Geometry: final body of the model. Coordinates: model frame, mm. Face numbers are marked on the shaded views. A direction names the side the tool comes from. Round coordinates to 2 decimals unless told otherwise and drop trailing zeros. Loops run counter-clockwise (first coordinate to the right, second up) from the corner with the lowest first, then second, coordinate; pieces in that order, holes last. Notation, with made-up numbers: (20.5, 51) - (54.5, 51) arc R23 ccw to (54.5, 71) - close; hole circle Ø9 at (-20.5, 60). An arc over 180 degrees is marked (long way). Answer in a Markdown table with one row per item. Add a question column.
from build123d import *

# Parameters (mm, degrees)
PAD_DEPTH         = 60
PAD_DEPTH_BACK    = 53
SKETCH001_R       = 11.1
SKETCH001_R_2     = 3.1
SKETCH001_R_3     = 1.6
SKETCH001_W       = 34.5
SKETCH001_H       = 60
POCKET_DEPTH      = 27.001
POCKET_DEPTH_BACK = -5.001
POCKET001_DEPTH   = 43.001
PAD001_DEPTH      = 5
PAD002_DEPTH      = 5
SKETCH005_W       = 43
SKETCH005_H       = 27
POCKET002_DEPTH   = 43.001
SKETCH006_W       = 5
SKETCH006_H       = 32
PAD003_DEPTH      = 15
SKETCH007_R       = 3.1
POCKET003_DEPTH   = 43.001
FILLET_R          = 2


with BuildPart() as part:
    # Sketch → Pad (new body, two sides)
    with BuildSketch(Plane.XZ) as pad_sk:
        Polygon((-43, 5), (27, 5), (27, 0), (0, 0), (0, -27), (-8.5, -27), (-8.5, 0), (-43, 0), align=None)
    extrude(amount=PAD_DEPTH)
    extrude(pad_sk.sketch, amount=-PAD_DEPTH_BACK)

    # Sketch001 → Pocket (cut, two sides)
    with BuildSketch(Plane.XY) as pocket_sk:
        with Locations((-22, 26.5)):
            Circle(SKETCH001_R)
        with Locations((15, 42)):
            Circle(SKETCH001_R_2)
        with Locations((15, -42)):
            Circle(SKETCH001_R_2)
        with Locations((15, 0)):
            Circle(SKETCH001_R_2)
        with Locations((-37.5, 42)):
            Circle(SKETCH001_R_3)
        with Locations((-6.5, 42)):
            Circle(SKETCH001_R_3)
        with Locations((-6.5, 11)):
            Circle(SKETCH001_R_3)
        with Locations((-37.5, 11)):
            Circle(SKETCH001_R_3)
        with Locations((-25.75, -30)):
            Rectangle(SKETCH001_W, SKETCH001_H)
    extrude(amount=-POCKET_DEPTH, mode=Mode.SUBTRACT)
    extrude(pocket_sk.sketch, amount=-POCKET_DEPTH_BACK, mode=Mode.SUBTRACT)

    # Sketch002 → Pocket001 (cut, through all)
    with BuildSketch(Plane.YZ):
        with BuildLine():
            ThreePointArc((-52.5, -11.9), (-55.6, -15), (-52.5, -18.1))
            Line((-52.5, -18.1), (-49.5, -18.1))
            ThreePointArc((-49.5, -18.1), (-46.4, -15), (-49.5, -11.9))
            Line((-52.5, -11.9), (-49.5, -11.9))
        make_face()
        with BuildLine():
            ThreePointArc((-10.5, -11.9), (-13.6, -15), (-10.5, -18.1))
            Line((-10.5, -18.1), (-7.5, -18.1))
            ThreePointArc((-7.5, -18.1), (-4.4, -15), (-7.5, -11.9))
            Line((-10.5, -11.9), (-7.5, -11.9))
        make_face()
    extrude(amount=-POCKET001_DEPTH, mode=Mode.SUBTRACT)

    # Sketch003 → Pad001 (join)
    with BuildSketch(Plane.XZ):
        Polygon((-43, 5), (-43, 0), (-8.5, -27), (0, -27), (0, 5), align=None)
    extrude(amount=-PAD001_DEPTH)

    # Sketch004 (on Face1 of Pad001) → Pad002 (join)
    with BuildSketch(Plane(origin=(0, 53, 0), x_dir=(1, 0, 0), z_dir=(0, 1, 0))):
        Polygon((-43, -5), (0, -5), (0, 27), (-8.5, 27), (-43, 0), align=None)
    extrude(amount=-PAD002_DEPTH)

    # Sketch005 → Pocket002 (cut, through all)
    with BuildSketch(Plane.YZ):
        with Locations((26.5, -13.5)):
            Rectangle(SKETCH005_W, SKETCH005_H)
    extrude(amount=-POCKET002_DEPTH, mode=Mode.SUBTRACT)

    # Sketch006 (on Face4 of Pocket002) → Pad003 (join)
    with BuildSketch(Plane(origin=(0, 53, 0), x_dir=(1, 0, 0), z_dir=(0, 1, 0))):
        with Locations((-2.5, 11)):
            Rectangle(SKETCH006_W, SKETCH006_H)
    extrude(amount=PAD003_DEPTH)

    # Sketch007 → Pocket003 (cut, through all)
    with BuildSketch(Plane.YZ):
        with Locations((60.5, -15)):
            Circle(SKETCH007_R)
    extrude(amount=-POCKET003_DEPTH, mode=Mode.SUBTRACT)

    # Fillet
    fillet_edges = [part.edges().sort_by_distance(p)[0] for p in [
        (27, -60, 2.5),
        (27, 53, 2.5),
        (-43, 0, 2.5),
        (-43, 53, 2.5),
    ]]
    fillet(fillet_edges, radius=FILLET_R)


solid = part.part
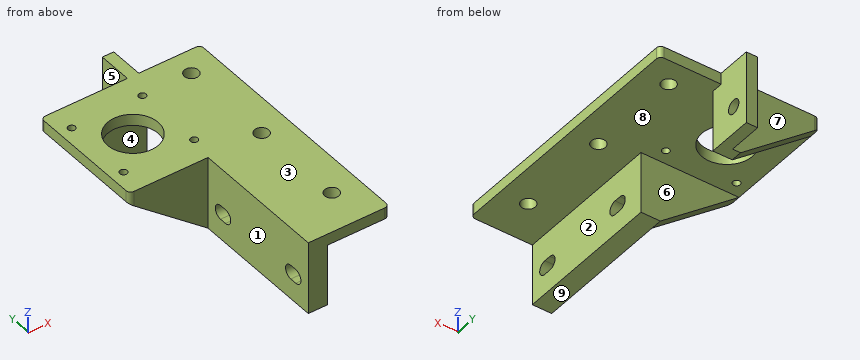
1) Contact query for flat-ended pins moving along their axis: pin 1 Ø9.5 at (x, z) = (-16.5, -18.5) entering from -Y; pin 2 Ø10 at (y, z) = (60.5, -15) entering from -X; pin 3 Ø6 at (y, z) = (59.5, -13) entering from +X. Output: stop coordinate, or through.
2) Section D-D, the plane y = 11. Return the cut outline in (x, z), and give its area (3 significant figures).
3) Section C-C, the plane x = -24.5. Return the cut outline in (y, z), and give its area (3 significant figures).
4) Material intervals for line 1 along Y through (x, z) = (15, 3); line 2 along Y through (x, z) = (-6.5, 2.85); line 3 along Y through (x, z) = (-37.5, 1.75), sorted ascending. Write a range as from..to.
5) Reachability of the marked faces 1, 2, 3, 4 and 5 from +Z, -Z, +X, -X, +Y, -Y: full face, straight path, thin tool, end or side. Return the list, or none.
6) Section B-B, the plane z = -15. Return the cut outline in (x, y).
7) Pull-direction query (Y, two-part tool) for the marked faces 6, 7, 8 and 9; classes: pulls with the +Y half, pulls with the -Y half, needs draft (parallel to the pull), parting line crosses it, or undercut.
8) Section A-A, the plane y = 26.5. Return the cut outline in (x, z), and give its area (3 significant figures).
Evaluation:
| question | item | result |
|---|---|---|
| 1 | pin 1 | stops at y = 0 |
| 1 | pin 2 | stops at x = -5 |
| 1 | pin 3 | stops at x = 0 |
| 2 | outline | (-43, 0) - (-39.1, 0) - (-39.1, 5) - (-43, 5) - close; (-35.9, 0) - (-8.1, 0) - (-8.1, 5) - (-35.9, 5) - close; (-4.9, 0) - (27, 0) - (27, 5) - (-4.9, 5) - close |
| 2 | area | 318 mm² |
| 3 | outline | (0, -14.48) - (5, -14.48) - (5, 0) - (15.69, 0) - (15.69, 5) - (0, 5) - close; (37.31, 0) - (48, 0) - (48, -14.48) - (53, -14.48) - (53, 5) - (37.31, 5) - close |
| 3 | area | 302 mm² |
| 4 | line 1 | y = -60..-45.1, -38.9..-3.1, 3.1..38.9, 45.1..53 |
| 4 | line 2 | y = -60..9.4, 12.6..40.4, 43.6..53 |
| 4 | line 3 | y = 0..9.4, 12.6..40.4, 43.6..53 |
| 5 | face 1 | +Z, -Z, -X, -Y |
| 5 | face 2 | -Z, +X, +Y, -Y |
| 5 | face 3 | +Z, +X, -X, +Y, -Y |
| 5 | face 4 | -Z, +X, -X |
| 5 | face 5 | +Z, -Z, -X, +Y |
| 6 | outline | (-23.83, 0) - (-8.5, 0) - (-8.5, -4.4) - (0, -4.4) - (0, 5) - (-23.83, 5) - close; (-23.83, 48) - (0, 48) - (0, 57.4) - (-5, 57.4) - (-5, 53) - (-23.83, 53) - close; (-8.5, -60) - (0, -60) - (0, -55.6) - (-8.5, -55.6) - close; (-8.5, -46.4) - (0, -46.4) - (0, -13.6) - (-8.5, -13.6) - close; (-5, 63.6) - (0, 63.6) - (0, 68) - (-5, 68) - close |
| 7 | face 6 | undercut |
| 7 | face 7 | pulls with the +Y half |
| 7 | face 8 | undercut |
| 7 | face 9 | needs draft |
| 8 | outline | (-43, 0) - (-33.1, 0) - (-33.1, 5) - (-43, 5) - close; (-10.9, 0) - (27, 0) - (27, 5) - (-10.9, 5) - close |
| 8 | area | 239 mm² |
